Here's how the part is built. I have some questions about the finished solid (model axes, mm). Face numbers are marked on the shaded views. Round coordinates to 2 decimals unless told otherwise and drop trailing zeros. Order: outer loops, then holes, each group sorted by start corner. A loop starts at its lowest first (then second) coordinate and runs counter-clockwise, first axis right, second up. Notation, with made-up numbers: M 77,53.5 L 110,53.5 A25 ccw 110,66.5 Z; hole C 11,56 d1. An arc over 180 degrees is marked long. Write item = value, one per line. Start each with the question number.
Item 1: I want a section at C-C, the plane z = 90. List the corners of the cut face in (x, y) for me, plus the area to 4 significant figures.
Item 2: I'm going to push flat-ended pins straight in: P1, Ø1, axis at y = 3, z = 85.5, coming from the -X side; P2, Ø0.8, axis at x = 0.5, z = 86, coming from the -Y side; P3, Ø0.5, axis at y = -0.5, z = 8, coming from the +X side; P4, Ø3, axis at y = 2, z = 60, coming from the +X side. Where does each tip first touch, or does it pass through?
Item 3: I want a section at A-A, the plane y = 2. List the corners of the cut face in (x, z) for me.
Item 4: Please list where these lines run through material, in increasing order: L1, parallel to Z at x = 11, y = 3.5; L2, parallel to Y at x = 2.5, z = 30; L3, parallel to Z at x = 3, y = 3.5.
Item 5: We'd pull the mould along Z, two halves only. Please class the marked faces 1, 2, 3 and 4: pulls with the +Z half, pulls with the -Z half, needs draft (parallel to the pull), parting line crosses it, or undercut.
Item 6: I want a section at B-B, the plane x = 2.5. List the corners of the cut face in (y, z) for me.
Item 7: I want a section at D-D, the plane z = 65.5. List the corners of the cut face in (x, y) for me, plus the area to 3 significant figures.
```python
from build123d import *

# Parameters (mm, degrees)
MAIN_DEPTH               = 120
ESQUISSE2_R              = 1.25
HOLESFORMOTORBOARD_DEPTH = 15.95
ESQUISSE4_R              = 1.6
HOLESFORMAKERBEAM_DEPTH  = 9
SKETCH1_W                = 100
SKETCH1_H                = 7
POWERBOARDPINHOLES_DEPTH = 7.45
SKETCH2_R                = 1.25
WINDOWFIXHOLES_DEPTH     = 15.95


with BuildPart() as part:
    # Esquisse1 → Main (new body)
    with BuildSketch(Plane.XY):
        Polygon((0, 7), (14.95, 7), (14.95, 0), (3.95, 0), (3.95, -1), (1.05, -1), (1.05, 0), (0, 0), align=None)
    extrude(amount=MAIN_DEPTH)

    # Esquisse2 → HolesForMotorBoard (cut, through all)
    with BuildSketch(Plane(origin=(14.95, 0, 0), x_dir=(0, 0, -1), z_dir=(1, 0, 0))):
        with Locations((-4.25, 5)):
            Circle(ESQUISSE2_R)
        with Locations((-115.75, 5)):
            Circle(ESQUISSE2_R)
    extrude(amount=-HOLESFORMOTORBOARD_DEPTH, mode=Mode.SUBTRACT)

    # Esquisse4 → HolesForMakerBeam (cut, through all)
    with BuildSketch(Plane(origin=(0, -1, 0), x_dir=(-1, 0, 0), z_dir=(0, -1, 0))):
        with Locations((-2.5, -100)):
            Circle(ESQUISSE4_R)
        with Locations((-2.5, -20)):
            Circle(ESQUISSE4_R)
    extrude(amount=-HOLESFORMAKERBEAM_DEPTH, mode=Mode.SUBTRACT)

    # Sketch1 → PowerBoardPinHoles (cut)
    with BuildSketch(Plane(origin=(14.95, 0, 0), x_dir=(0, 0, -1), z_dir=(1, 0, 0))):
        with Locations((-60, 3.5)):
            Rectangle(SKETCH1_W, SKETCH1_H)
    extrude(amount=-POWERBOARDPINHOLES_DEPTH, mode=Mode.SUBTRACT)

    # Sketch2 → WindowFixHoles (cut, through all)
    with BuildSketch(Plane.ZY):
        with Locations((60, 2)):
            Circle(SKETCH2_R)
        with Locations((30, 2)):
            Circle(SKETCH2_R)
        with Locations((90, 2)):
            Circle(SKETCH2_R)
    extrude(amount=-WINDOWFIXHOLES_DEPTH, mode=Mode.SUBTRACT)


solid = part.part
```
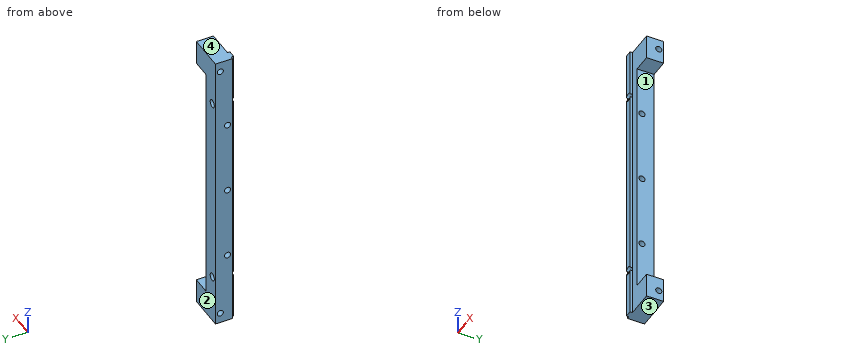
Filled in:
q1.outline = M 0,0 L 1.05,0 L 1.05,-1 L 3.95,-1 L 3.95,0 L 7.5,0 L 7.5,0.75 L 0,0.75 Z; M 0,3.25 L 7.5,3.25 L 7.5,7 L 0,7 Z
q1.area = 36.65 mm^2
q2.P1 = 0
q2.P2 = 0
q2.P3 = 3.95
q2.P4 = 7.5
q3.outline = M 0,0 L 14.95,0 L 14.95,10 L 7.5,10 L 7.5,28.75 L 0,28.75 Z; M 0,31.25 L 7.5,31.25 L 7.5,58.75 L 0,58.75 Z; M 0,61.25 L 7.5,61.25 L 7.5,88.75 L 0,88.75 Z; M 0,91.25 L 7.5,91.25 L 7.5,110 L 14.95,110 L 14.95,120 L 0,120 Z; hole C 2.5,20 d3.2; hole C 2.5,100 d3.2
q4.L1 = 0 to 10, 110 to 120
q4.L2 = -1 to 0.75, 3.25 to 7
q4.L3 = 0 to 18.48, 21.52 to 98.48, 101.52 to 120
q5.face_1 = undercut
q5.face_2 = needs draft
q5.face_3 = pulls with the -Z half
q5.face_4 = pulls with the +Z half
q6.outline = M -1,0 L 7,0 L 7,18.4 L -1,18.4 Z; M -1,21.6 L 7,21.6 L 7,98.4 L -1,98.4 Z; M -1,101.6 L 7,101.6 L 7,120 L -1,120 Z; hole C 2,30 d2.5; hole C 2,60 d2.5; hole C 2,90 d2.5; hole C 5,4.25 d2.5; hole C 5,115.75 d2.5
q7.outline = M 0,0 L 1.05,0 L 1.05,-1 L 3.95,-1 L 3.95,0 L 7.5,0 L 7.5,7 L 0,7 Z
q7.area = 55.4 mm^2
